```python
from build123d import *

# Parameters (mm, degrees)
F0_W     = 101.6
F0_H     = 50.8
F1_DEPTH = 12.7
F2_R     = 3.4925
F3_DEPTH = 6.35


with BuildPart() as f1:
    # F0 (on Top) → F1 (new body)
    with BuildSketch(Plane.XY):
        with Locations((1.517599, 0.191483)):
            Rectangle(F0_W, F0_H)
    extrude(amount=-F1_DEPTH)

    # F2 (on Top) → F3 (cut)
    with BuildSketch(Plane.XY):
        with BuildLine():
            Line((8.705417, 2.137989), (9.813658, 4.354471))
            ThreePointArc((9.813658, 4.354471), (-1.02506, 21.350936), (-10.887856, 3.770183))
            Line((-10.887856, 3.770183), (-11.883179, 4.267844))
            ThreePointArc((-11.883179, 4.267844), (-27.596218, -11.587781), (-5.542731, -8.13175))
            Line((-5.542731, -8.13175), (11.687214, -16.746723))
            ThreePointArc((11.687214, -16.746723), (28.544601, -4.407269), (8.705417, 2.137989))
        make_face()
        with Locations((-17.136821, -6.239439)):
            Circle(F2_R, mode=Mode.SUBTRACT)
        with BuildLine():
            Line((12.397165, -15.326819), (-14.864975, -1.695749))
            ThreePointArc((-14.864975, -1.695749), (-21.019695, -9.515059), (-12.27537, -4.765431))
            Line((-12.27537, -4.765431), (-7.041321, -7.382455))
            ThreePointArc((-7.041321, -7.382455), (-26.066643, -11.085456), (-12.59313, 2.847941))
            Line((-12.59313, 2.847941), (-1.233905, -2.831672))
            Line((-1.233905, -2.831672), (3.850064, 7.336267))
            ThreePointArc((3.850064, 7.336267), (-3.969246, 13.490986), (0.780383, 4.746662))
            Line((0.780383, 4.746662), (-1.836642, -0.487387))
            ThreePointArc((-1.836642, -0.487387), (-5.539642, 18.537934), (8.393754, 5.064422))
            Line((8.393754, 5.064422), (3.309785, -5.103517))
            Line((3.309785, -5.103517), (14.66901, -10.783129))
            ThreePointArc((14.66901, -10.783129), (20.82373, -2.963819), (12.079405, -7.713448))
            Line((12.079405, -7.713448), (6.845356, -5.096423))
            ThreePointArc((6.845356, -5.096423), (25.870677, -1.393423), (12.397165, -15.326819))
        make_face(mode=Mode.SUBTRACT)
        with Locations((16.940855, -6.239439)):
            Circle(F2_R, mode=Mode.SUBTRACT)
        with Locations((-0.693626, 9.608112)):
            Circle(F2_R, mode=Mode.SUBTRACT)
    extrude(amount=-F3_DEPTH, mode=Mode.SUBTRACT)


solid = f1.part
```
The listing builds one solid part. Answer for the finished solid, in the listing's coordinates (mm). A direction names the side the tool comes from. Coordinates: 2 decimals unless noted, no trailing zeros. Loops run counter-clockwise (first coordinate to the right, second up) from the corner with the lowest first, then second, coordinate; pieces in that order, holes last. Notation, with made-up numbers: M 20.5,-30 L 58.5,-30 A26 cw 58.5,-14 Z; hole C 3,27.5 d3. An arc over 180 degrees is marked long. Answer as CSV lines item,"result". Start each with the question number.
(1) Find the intervals of material crossed by L1, parallel to X at y = 10, z = -6; L2, parallel to X at y = 9, z = -6; L3, parallel to Y at x = -16.5, z = -0.5, in increasing order. Write a range as [from, to].
(2) The part is cut by section C-C (y = 17.5). Give the vertices of the cut face in (x, z), and give its area (3 significant figures).
(3) The part is cut by section A-A (z = -1). Give the vertices of the cut face in (x, y) (1 decimal), and give its area (3 significant figures).
(4) For faces 1 (the flat face through (12, 6, 0)), 2 (the cylindrical face through (28.6, -4.8, -3.1)), determine the directions among +Z, -Z, +X, -X, +Y, -Y from which every point of the face is accessible in a straight line to the end or side of a thin tool.
(5) The part is cut by section B-B (x = -25). Give the vertices of the cut face in (y, z).
(6) The mould has two halves that part along Y. Classify faces 3 (the flat face through (1, 1, -12.7)), 4 (the flat face through (1, -25.209, -6)), 5 (the cylindrical face through (-5.853, 18.361, -3.131)): pulls with the +Y half, pulls with the -Y half, needs draft (parallel to the pull), parting line crosses it, or undercut.
Determined:
1,L1,"[-49.28, -12.43], [-10.85, -5.76], [-4.16, 2.78], [4.37, 9.46], [11.05, 52.32]"
1,L2,"[-49.28, -12.43], [-10.84, -5.74], [-4.13, 2.75], [4.35, 9.45], [11.04, 52.32]"
1,L3,"[-25.21, -17.97], [-16.38, -11.28], [-9.67, -2.81], [-1.2, 3.9], [5.49, 25.59]"
2,outline,"M -49.28,-12.7 L 52.32,-12.7 L 52.32,0 L 8.01,0 L 8.01,-6.35 L 5.71,-6.35 L 5.71,0 L -7.09,0 L -7.09,-6.35 L -9.4,-6.35 L -9.4,0 L -49.28,0 Z"
2,area,"1,260 mm2"
3,outline,"M -49.3,-25.2 L 52.3,-25.2 L 52.3,25.6 L -49.3,25.6 Z; C -17.1,-6.2 d7; M -14.9,-1.7 L 12.4,-15.3 A10.2 ccw long 6.8,-5.1 L 12.1,-7.7 A5.1 cw long 14.7,-10.8 L 3.3,-5.1 L 8.4,5.1 A10.2 ccw long -1.8,-0.5 L 0.8,4.7 A5.1 cw long 3.9,7.3 L -1.2,-2.8 L -12.6,2.8 A10.2 ccw long -7,-7.4 L -12.3,-4.8 A5.1 cw long Z; C -0.7,9.6 d7; C 16.9,-6.2 d7; hole M -11.9,4.3 A11.7 ccw long -5.5,-8.1 L 11.7,-16.7 A11.7 ccw long 8.7,2.1 L 9.8,4.4 A11.7 ccw long -10.9,3.8 Z"
3,area,"4,680 mm2"
4,face 1,"+Z, +X, -X, +Y, -Y"
4,face 2,"+Z"
5,outline,"M -25.21,-12.7 L 25.59,-12.7 L 25.59,0 L 2.49,0 L 2.49,-6.35 L 0.19,-6.35 L 0.19,0 L -12.67,0 L -12.67,-6.35 L -14.97,-6.35 L -14.97,0 L -25.21,0 Z"
6,face 3,"needs draft"
6,face 4,"pulls with the -Y half"
6,face 5,"undercut"
